from build123d import *

# Parameters (mm, degrees)
SKETCH1_W           = 36
SKETCH1_H           = 10
BOSS_EXTRUDE1_DEPTH = 12
SKETCH2_W           = 14
SKETCH2_H           = 12
BOSS_EXTRUDE2_DEPTH = 19
SKETCH3_R           = 2.25
CUT_EXTRUDE1_DEPTH  = 11
SKETCH4_R           = 4
CUT_EXTRUDE2_DEPTH  = 4
M6_TAPPED_HOLE1_D   = 5


with BuildPart() as part:
    # Sketch1 → Boss-Extrude1 (new body)
    with BuildSketch(Plane.XY):
        with Locations((9.722605043, -1.956268222)):
            Rectangle(SKETCH1_W, SKETCH1_H)
    extrude(amount=BOSS_EXTRUDE1_DEPTH)

    # Sketch2 → Boss-Extrude2 (add)
    with BuildSketch(Plane(origin=(0, 3.043731778, 0), x_dir=(1, 0, 0), z_dir=(0, 1, 0))):
        with Locations((20.722605043, -6)):
            Rectangle(SKETCH2_W, SKETCH2_H)
    extrude(amount=BOSS_EXTRUDE2_DEPTH)

    # Sketch3 → Cut-Extrude1 (cut, through all)
    with BuildSketch(Plane(origin=(0, 3.043731778, 0), x_dir=(1, 0, 0), z_dir=(0, 1, 0))):
        with Locations((-3.277394957, -6)):
            Circle(SKETCH3_R)
        with Locations((8.722605043, -6)):
            Circle(SKETCH3_R)
    extrude(amount=-CUT_EXTRUDE1_DEPTH, mode=Mode.SUBTRACT)

    # Sketch4 → Cut-Extrude2 (cut)
    with BuildSketch(Plane(origin=(0, 3.043731778, 0), x_dir=(1, 0, 0), z_dir=(0, 1, 0))):
        with Locations((-3.277394957, -6)):
            Circle(SKETCH4_R)
        with Locations((8.722605043, -6)):
            Circle(SKETCH4_R)
    extrude(amount=-CUT_EXTRUDE2_DEPTH, mode=Mode.SUBTRACT)

    # M6 Tapped Hole1 (through all)
    with Locations(Plane(origin=(27.722605043, 0, 0), x_dir=(0, 0, -1), z_dir=(1, 0, 0))):
        with Locations((-6, 16.043731778)):
            Hole(M6_TAPPED_HOLE1_D / 2)


solid = part.part
Input: part model. Units: mm. Frame: model coordinates. A direction names the side the tool comes from. Give positions to 0.01 mm unless a question says otherwise; leave off trailing zeros. Order: outer loops, then holes, each group sorted by start corner. A loop starts at its lowest first (then second) coordinate and runs counter-clockwise, first axis right, second up. Notation, with made-up numbers: (75, -8) - (119, -8) arc R17 ccw to (119, 1) - close; hole circle Ø8 at (44, 88.5). An arc over 180 degrees is marked (long way). Answer as a JSON object with one key per item and string values. Group by question number.
Q1. Line query: probe 1 along X at (y, z) = (1.4, 6); probe 2 along X at (y, z) = (-2.5, 6); probe 3 along Y at (x, z) = (22.5, 6). Output: solid intervals per line, ascending.
Q2. Mould query, pull axis Z, two halves, no side actions, for faces 4 (the face through (3, 3.044, 6)), 5 (the face through (13, 1, 0)), 6 (the face through (10.44, -0.956, 7.72)). Classes: pulls with the +Z half, pulls with the -Z half, needs draft (parallel to the pull), parting line crosses it, or undercut.
Q3. Cut plane D-D, the plane y = -0.5. Output: boundary loops of the cut face in (x, z), then the cut area to 3 significant figures.
Q4. Cut plane B-B, the plane y = 17.5. Output: boundary loops of the cut face in (x, z), then the cut area to 3 significant figures.
Q5. Cut plane A-A, the plane z = 6. Output: boundary loops of the cut face in (x, y), then the cut area to 3 significant figures.
Q6. First-contact query: pin 1 Ø3.5 at (x, z) = (8.72, 6) entering from -Y; pin 2 Ø5 at (x, z) = (-3.28, 6) entering from +Y; pin 3 Ø3.5 at (x, z) = (2, 5.5) entering from +Y; pin 4 Ø3.5 at (y, z) = (12, 6.5) entering from -X. Flat tips, straight axial feed; report the tip coordinate or a pass-through.
Q7. Cut plane C-C, the plane x = -5. Output: boundary loops of the cut face in (y, z), then the cut area to 4 significant figures.
Q8. Set-up query: faces 1 (the face through (13.723, 12, 6)), 2 (the face through (-4.145, 1.072, 9.905)), 3 (the face through (10.869, -3.914, 5.324)). Return all of +Z, -Z, +X, -X, +Y, -Y with unobstructed straight access to the full face (end or side cutting, diameter ignored); none if empty.
Results:
{
 "1": {"probe 1": "-8.28 to -7.28, 0.72 to 4.72, 12.72 to 27.72", "probe 2": "-8.28 to -5.53, -1.03 to 6.47, 10.97 to 27.72", "probe 3": "-6.96 to 13.54, 18.54 to 22.04"},
 "2": {"face 4": "needs draft", "face 5": "pulls with the -Z half", "face 6": "undercut"},
 "3": {"outline": "(-8.28, 0) - (27.72, 0) - (27.72, 12) - (-8.28, 12) - close; hole circle Ø8 at (-3.28, 6); hole circle Ø8 at (8.72, 6)", "area": "331 mm^2"},
 "4": {"outline": "(13.72, 0) - (27.72, 0) - (27.72, 3.97) - (13.72, 3.97) - close; (13.72, 8.03) - (27.72, 8.03) - (27.72, 12) - (13.72, 12) - close", "area": "111 mm^2"},
 "5": {"outline": "(-8.28, -6.96) - (-5.53, -6.96) - (-5.53, -0.96) - (-7.28, -0.96) - (-7.28, 3.04) - (-8.28, 3.04) - close; (-1.03, -6.96) - (6.47, -6.96) - (6.47, -0.96) - (4.72, -0.96) - (4.72, 3.04) - (0.72, 3.04) - (0.72, -0.96) - (-1.03, -0.96) - close; (10.97, -6.96) - (27.72, -6.96) - (27.72, 13.54) - (13.72, 13.54) - (13.72, 3.04) - (12.72, 3.04) - (12.72, -0.96) - (10.97, -0.96) - close; (13.72, 18.54) - (27.72, 18.54) - (27.72, 22.04) - (13.72, 22.04) - close", "area": "438 mm^2"},
 "6": {"pin 1": "through", "pin 2": "y = -0.96", "pin 3": "y = 3.04", "pin 4": "x = 13.72"},
 "7": {"outline": "(-6.96, 0) - (3.04, 0) - (3.04, 2.39) - (-0.96, 2.39) - (-0.96, 4.55) - (-6.96, 4.55) - close; (-6.96, 7.45) - (-0.96, 7.45) - (-0.96, 9.61) - (3.04, 9.61) - (3.04, 12) - (-6.96, 12) - close", "area": "73.75 mm^2"},
 "8": {"face 1": "+Z, -Z, -X, +Y", "face 2": "+Y", "face 3": "+Y, -Y"}
}
